from build123d import *

# Parameters (mm, degrees)
STOCK_TEATHERED_START                        = 85.075
STOCK_TEATHERED_SWERVE_OUTER_MODUAL_1_OU_R   = 2.0193
STOCK_TEATHERED_SWERVE_OUTER_MODUAL_1_OU_R_2 = 4.7625
STOCK_TEATHERED_SWERVE_OUTER_MODUAL_1_DEPTH  = 3.175
CHAMFER1_SIZE                                = 0.635


# Read off the part's stored shape, not the designer's step: Stock-Teathered Swerve Outer Modual-1
with BuildPart() as part:
    # Stock-Teathered Swerve Outer Modual-1 ou → Stock-Teathered Swerve Outer Modual-1 (new body)
    with BuildSketch(Plane(origin=(0, 0, 0), x_dir=(1, 0, 0), z_dir=(0, 1, 0)).offset(STOCK_TEATHERED_START)):
        with BuildLine():
            ThreePointArc((69.17405827, 6.398212246), (74.59793655, 11.484662283), (68.44777711, 15.663892887))
            ThreePointArc((68.44777711, 15.663892887), (43.031292772, 16.425853008), (23.381787081, 32.565096654))
            ThreePointArc((23.381787081, 32.565096654), (16.469460575, 33.864059213), (15.801303162, 26.862550296))
            ThreePointArc((15.801303162, 26.862550296), (26.644984318, 4.602603852), (23.897134883, -20.005117705))
            ThreePointArc((23.897134883, -20.005117705), (27.16089255, -26.456318028), (33.039902775, -22.248309176))
            ThreePointArc((33.039902775, -22.248309176), (44.943402215, -0.150432703), (69.17405827, 6.398212246))
        make_face()
        with Locations((28.295721181, -21.830999635)):
            Circle(STOCK_TEATHERED_SWERVE_OUTER_MODUAL_1_OU_R, mode=Mode.SUBTRACT)
        with Locations((38.300729341, 9.113233891)):
            Circle(STOCK_TEATHERED_SWERVE_OUTER_MODUAL_1_OU_R_2, mode=Mode.SUBTRACT)
        with Locations((19.332478919, 30.058204223)):
            Circle(STOCK_TEATHERED_SWERVE_OUTER_MODUAL_1_OU_R, mode=Mode.SUBTRACT)
        with Locations((69.85, 11.1125)):
            Circle(STOCK_TEATHERED_SWERVE_OUTER_MODUAL_1_OU_R, mode=Mode.SUBTRACT)
    extrude(amount=STOCK_TEATHERED_SWERVE_OUTER_MODUAL_1_DEPTH)

    # Chamfer1
    chamfer1_edges = [part.edges().sort_by_distance(p)[0] for p in [
        (26.644984318, 88.25, -4.602603852),
        (27.16089255, 88.25, 26.456318028),
        (33.538229341, 85.075, -9.113233891),
        (33.538229341, 88.25, -9.113233891),
        (26.276421181, 85.075, 21.830999635),
        (44.943402215, 88.25, 0.150432703),
        (26.276421181, 88.25, 21.830999635),
        (67.8307, 85.075, -11.1125),
        (74.59793655, 88.25, -11.484662283),
        (67.8307, 88.25, -11.1125),
        (17.313178919, 85.075, -30.058204223),
        (17.313178919, 88.25, -30.058204223),
        (43.031292772, 88.25, -16.425853008),
        (74.59793655, 85.075, -11.484662283),
        (44.943402215, 85.075, 0.150432703),
        (27.16089255, 85.075, 26.456318028),
        (26.644984318, 85.075, -4.602603852),
        (16.469460575, 85.075, -33.864059213),
        (43.031292772, 85.075, -16.425853008),
        (16.469460575, 88.25, -33.864059213),
    ]]
    chamfer(chamfer1_edges, length=CHAMFER1_SIZE)


solid = part.part
Verification items for the finished model (mm, model axes). Coordinates: 2 decimals unless noted, no trailing zeros. Answer as a JSON object with one key per item and string values. Group by question number.
Item 1: Scan lines: probe 1 along X at (y, z) = (87.4, -10.5); probe 2 along X at (y, z) = (85.75, -11.5); probe 3 along X at (y, z) = (85.25, 20). Record each from-to range of solid material in increasing order.
Item 2: Mould release check, pull along Z, two halves, no side actions. Record for faces 1 (the cylindrical face through (44.66, 86.65, 0.38)), 2 (the flat face through (36, 88.25, -4)), 3 (the conical face through (71, 88, -9)): +Z half, -Z half, draft (parallel to the pull), parting line (faces both ways), or undercut.
Item 3: Depth check by flat-ended pin: pin 1 (7.5 mm diameter, centred on x = 38.3, z = -9.11, fed in from +Y); pin 2 (1.5 mm diameter, centred on x = 48, y = 86.5, fed in from +Z); pin 3 (1 mm diameter, centred on y = 87, z = 1.5, fed in from +X); pin 4 (1 mm diameter, centred on x = 30, y = 85.5, fed in from -Z). Enter the tip coordinate at first touch or a pass-through.
Evaluation:
{
 "1": {"probe 1": "x = 25.21 to 33.74, 42.86 to 67.93, 71.77 to 74.57", "probe 2": "x = 24.87 to 34.18, 42.42 to 67.87, 71.83 to 74.6", "probe 3": "x = 24.4 to 26.62, 29.97 to 32.85"},
 "2": {"face 1": "+Z half", "face 2": "draft", "face 3": "undercut"},
 "3": {"pin 1": "passes through", "pin 2": "stops at z = -1.52", "pin 3": "stops at x = 43.92", "pin 4": "stops at z = -24.93"}
}
